Input: dimensioned drawing with shaded views. Units: mm. Origin: part minimum x, y, z. A direction names the side the tool comes from. Give positions to 0.01 mm unless a question says otherwise; leave off trailing zeros.
Q1. Reachability of the marked faces 1 and 2 from +Z, -Z, +X, -X, +Y, -Y: full face, straight path, thin tool, end or side. Return the list, or none.
Q2. Line query: line 1 (Z direction, x = 6.35, y = 2.2); line 2 (X direction, y = 8.5, z = 2) (1 decimal); line 3 (X direction, y = 9.25, z = 8) (1 decimal). Output: solid intervals per line, ascending.
Q3. Pin query (flat end, axial travel): pin 1 Ø4 at (y, z) = (16.5, 10) entering from -X; pin 2 Ø3 at (y, z) = (8.5, 5.5) entering from -X; pin 3 Ø3 at (y, z) = (13.5, 5) entering from +X. Return the tip coordinate at first contact, or that it passes through.
Q4. Section A-A (z = 7.25). State how many separate pieces and enclosed holes the cut face has, plus the area to 3 significant figures.
Q5. Mould query, pull axis Z, two halves, no side actions, for the marked faces 3, 4 and 5. Classes: +Z half, -Z half, draft (parallel to the pull), parting line (faces both ways), or undercut.
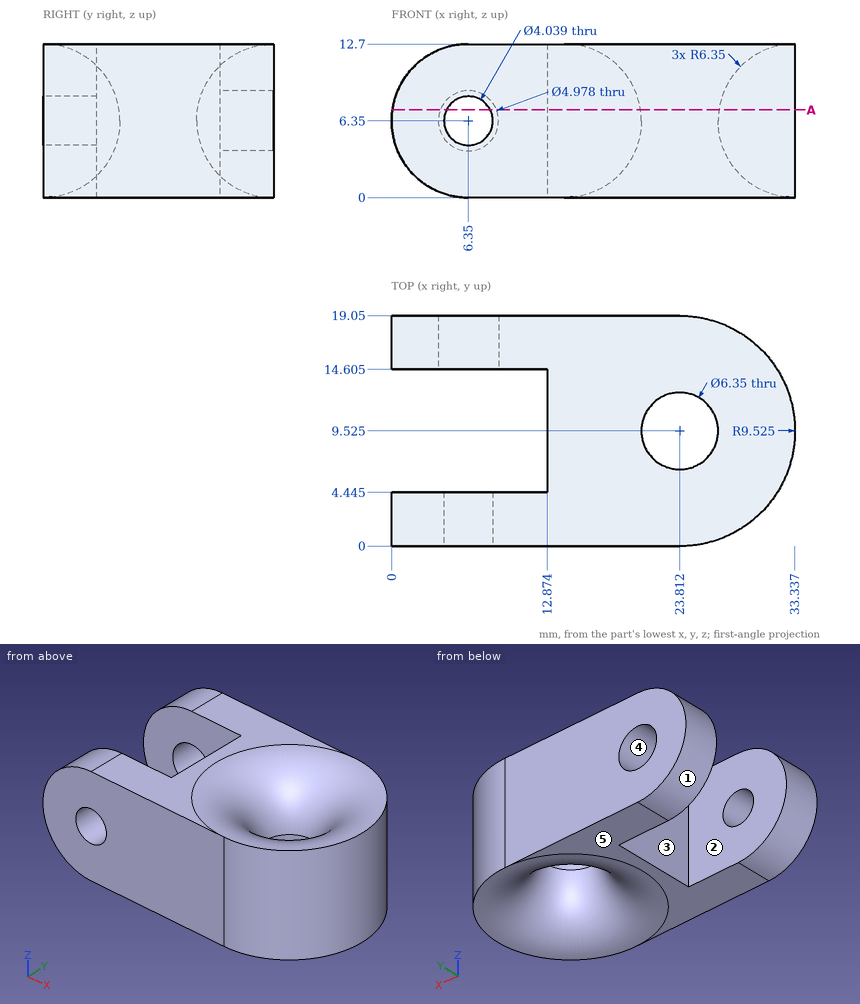
Computed:
1. face 1: -X, +Y, -Y
1. face 2: +Z, -Z, -X
2. line 1: z = 0 to 4.33, 8.37 to 12.7
2. line 2: x = 12.9 to 19, 28.6 to 33.3
2. line 3: x = 12.9 to 20.4, 27.2 to 33.3
3. pin 1: stops at x = 0.22
3. pin 2: stops at x = 12.87
3. pin 3: stops at x = 33.01
4. separate pieces: 3
4. enclosed holes: 1
4. area: 395 mm2
5. face 3: draft
5. face 4: undercut
5. face 5: -Z half
